Work out the finished part from the listing and answer in its coordinate system (mm). Face numbers are marked on the shaded views. A direction names the side the tool comes from. Round coordinates to 2 decimals unless told otherwise and drop trailing zeros. Order: outer loops, then holes, each group sorted by start corner. A loop starts at its lowest first (then second) coordinate and runs counter-clockwise, first axis right, second up. Notation, with made-up numbers: (47.5, 86) - (91.5, 86) arc R14 cw to (91.5, 103) - close; hole circle Ø5 at (44.25, 47). An arc over 180 degrees is marked (long way). Put each result on its own line as item: value.
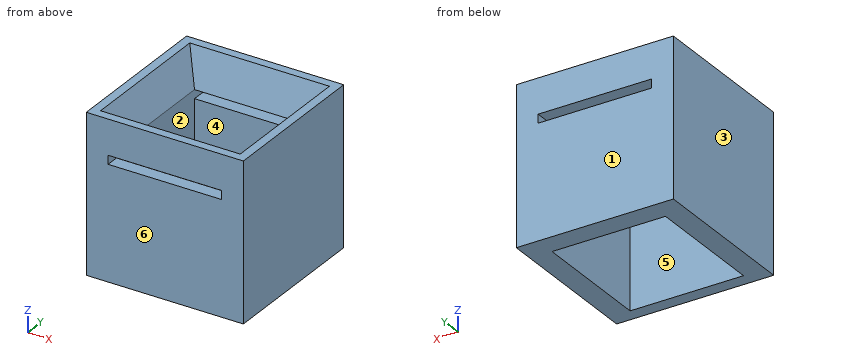
```python
from build123d import *

# Parameters (mm, degrees)
SKETCH1_W               = 457.2
SKETCH1_H               = 457.2
BOSS_EXTRUDE1_DEPTH     = 457.2
SKETCH4_W               = 330.2
SKETCH4_H               = 330.2
CUT_EXTRUDE1_DEPTH      = 457.2
SKETCH5_W               = 330.2
SKETCH5_H               = 355.6
CUT_EXTRUDE2_DEPTH      = 25.4
CUT_EXTRUDE3_DEPTH      = 792.893629278
CUT_EXTRUDE3_DEPTH_BACK = 792.893629278
SKETCH7_W               = 330.2
SKETCH7_H               = 25.4


with BuildPart() as part:
    # Sketch1 → Boss-Extrude1 (new body)
    with BuildSketch(Plane.XY):
        with Locations((228.6, 228.6)):
            Rectangle(SKETCH1_W, SKETCH1_H)
    extrude(amount=BOSS_EXTRUDE1_DEPTH)

    # Sketch2 → Cut-Loft1 section 0
    with BuildSketch(Plane.XY.offset(457.2)):
        with BuildLine():
            Line((25.4, 25.4), (431.8, 25.4))
            Line((431.8, 25.4), (431.8, 431.8))
            Line((431.8, 431.8), (25.4, 431.8))
            Line((25.4, 431.8), (25.4, 25.4))
        make_face()
    # Sketch3 → Cut-Loft1 section 1
    with BuildSketch(Plane.XY.offset(355.6)):
        with BuildLine():
            Line((63.5, 63.5), (393.7, 63.5))
            Line((393.7, 63.5), (393.7, 393.7))
            Line((393.7, 393.7), (63.5, 393.7))
            Line((63.5, 393.7), (63.5, 63.5))
        make_face()
    loft(mode=Mode.SUBTRACT)

    # Sketch4 → Cut-Extrude1 (cut)
    with BuildSketch(Plane.XY.offset(355.6)):
        with Locations((228.6, 228.6)):
            Rectangle(SKETCH4_W, SKETCH4_H)
    extrude(amount=-CUT_EXTRUDE1_DEPTH, mode=Mode.SUBTRACT)

    # Sketch5 → Cut-Extrude2 (cut)
    with BuildSketch(Plane(origin=(0, 63.5, 0), x_dir=(1, 0, 0), z_dir=(0, 1, 0))):
        with Locations((228.6, -177.8)):
            Rectangle(SKETCH5_W, SKETCH5_H)
    extrude(amount=-CUT_EXTRUDE2_DEPTH, mode=Mode.SUBTRACT)

    # Sketch7 → Cut-Extrude3 (cut, two sides: drawn at the far end of the back side and taken through both)
    with BuildSketch(Plane(origin=(0, 457.2, 0), x_dir=(1, 0, 0), z_dir=(0, 1, 0)).offset(-CUT_EXTRUDE3_DEPTH_BACK)):
        with Locations((228.6, -342.9)):
            Rectangle(SKETCH7_W, SKETCH7_H)
    extrude(amount=CUT_EXTRUDE3_DEPTH + CUT_EXTRUDE3_DEPTH_BACK, mode=Mode.SUBTRACT)


solid = part.part
```
1) For a pull along Y with two mould halves and no side action, classify the marked faces 1, 2 and 3 as pulls with the +Y half, pulls with the -Y half, needs draft (parallel to the pull), parting line crosses it, or undercut.
Findings below:
face 1: pulls with the +Y half
face 2: undercut
face 3: needs draft
2) A cutting plane is placed at B-B on x = 120. Give the number of separate pieces and of enclosed holes in the cut face, then the cut area to 3 significant figures.
Findings below:
separate pieces: 4
enclosed holes: 0
area: 42,600 mm2
3) A cutting plane is placed at A-A on z = 217. Write down the section's boundary in (x, y), then the cut area to 3 significant figures.
Findings below:
outline: (0, 0) - (457.2, 0) - (457.2, 457.2) - (0, 457.2) - close; hole (63.5, 38.1) - (393.7, 38.1) - (393.7, 393.7) - (63.5, 393.7) - close
area: 91,600 mm2
4) Straight lines are drawn through the part: L1, parallel to Y at x = 325.5, z = 146; L2, parallel to Z at x = 307.5, y = 432; L3, parallel to X at y = 214.5, z = 123. For each, find the intervals that lie inside material, in ascending order. Write a range as from..to.
Findings below:
L1: y = 0..38.1, 393.7..457.2
L2: z = 0..330.2, 355.6..457.2
L3: x = 0..63.5, 393.7..457.2
5) For the marked faces 4, 5 and 6, determine the directions among +Z, -Z, +X, -X, +Y, -Y from which every point of the face is accessible in a straight line to the end or side of a thin tool.
Findings below:
face 4: +Z, -Z
face 5: -Z
face 6: +Z, -Z, +X, -X, -Y
